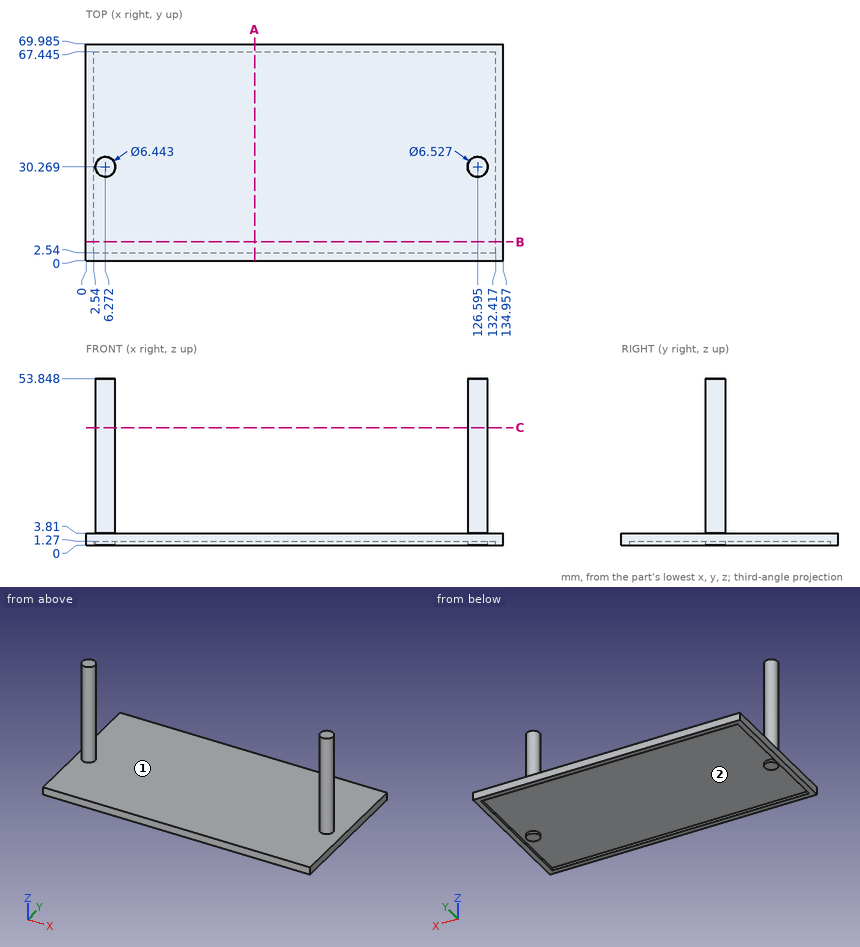
Here's the drawing with two shaded views (mm, measured from the low corner). I have some questions. Round coordinates to 2 decimals unless told otherwise and drop trailing zeros. Order: outer loops, then holes, each group sorted by start corner. A loop starts at its lowest first (then second) coordinate and runs counter-clockwise, first axis right, second up. Notation, with made-up numbers: M 53,-19 L 57,-19 A30 cw 57,9 Z; hole C -32.75,-32.75 d5. An arc over 180 degrees is marked long. Answer in a Markdown table with one row per item.
Item 1: Imagine slicing it at B-B, the plane y = 6. Write out the boundary of the cut face in (x, z), and give its area (3 significant figures).
A:
| item | result |
|---|---|
| outline | M 0,0 L 2.54,0 L 2.54,1.27 L 132.42,1.27 L 132.42,0 L 134.96,0 L 134.96,3.81 L 0,3.81 Z |
| area | 349 mm2 |
Item 2: Imagine slicing it at C-C, the plane z = 38. Write out the boundary of the cut face in (x, y) (1 decimal).
A:
| item | result |
|---|---|
| outline | C 6.3,30.3 d6.4; C 126.6,30.3 d6.5 |
Item 3: If I drill on L1, parallel to Z at x = 84.5, y = 18.5; L2, parallel to Y at x = 6, z = 9.5, over which ranges is the centre line in solid material (lowest first)? Write a range as from..to.
A:
| item | result |
|---|---|
| L1 | z = 1.27..3.81 |
| L2 | y = 27.06..33.48 |
Item 4: I'm going to push flat-ended pins straight in: pin 1 (10 mm diameter, centred on x = 30, y = 61, fed in from +Z); pin 2 (8 mm diameter, centred on x = 97.5, y = 40, fed in from -Z); pin 3 (1 mm diameter, centred on y = 21.5, z = 0.5, fed in from -X); pin 4 (4 mm diameter, centred on y = 28.5, z = 22, fed in from +X). Where does each tip first touch, or does it pass through?
A:
| item | result |
|---|---|
| pin 1 | stops at z = 3.81 |
| pin 2 | stops at z = 1.27 |
| pin 3 | stops at x = 0 |
| pin 4 | stops at x = 129.86 |
Item 5: Thinking about a two-plate mould opening in Y: for the marked faces 1 and 2, which applies, +Y half, -Y half, draft (parallel to the pull), parting line (faces both ways), or undercut?
A:
| item | result |
|---|---|
| face 1 | draft |
| face 2 | undercut |
Item 6: Imagine slicing it at A-A, the plane x = 54.5. Write out the boundary of the cut face in (y, z) (1 decimal), and give its area (3 significant figures).
A:
| item | result |
|---|---|
| outline | M 0,0 L 2.5,0 L 2.5,1.3 L 67.4,1.3 L 67.4,0 L 70,0 L 70,3.8 L 0,3.8 Z |
| area | 184 mm2 |
